Check sheet for the modelled part. Datum: model origin and axes. Units: mm. Give positions to 0.01 mm unless a question says otherwise; leave off trailing zeros. Order: outer loops, then holes, each group sorted by start corner. A loop starts at its lowest first (then second) coordinate and runs counter-clockwise, first axis right, second up. Notation, with made-up numbers: (22, 3) -> (40, 3) arc R19 ccw to (40, 37) -> close; hole circle Ø1 at (61.25, 88). An arc over 180 degrees is marked (long way). Answer in a Markdown table with one row per item. Add a question column.
(1) Cross-section at B-B (x = 4.75). Record the cut outline in (y, z), then the cut area to 3 significant figures.
(2) Thickness scan on L1, parallel to Y at x = 6, z = 3.75; L2, parallel to Z at x = -1.75, y = 1.85; L3, parallel to Z at x = -1.5, y = 2.9. Record the ranges inside material, lowest first. Write a range as [from, to].
(3) Cross-section at A-A (y = 4.15). Record the cut outline in (x, z).
(4) Go/stop test with flat-tipped pins: pin 1 (5 mm diameter, centred on x = 0, z = 4, fed in from -Y); pin 2 (1 mm diameter, centred on x = 1.5, y = 2, fed in from -Z); pin 3 (1.5 mm diameter, centred on x = 0.5, z = -4.5, fed in from -Y). Record where each tip stops, or that it passes through.
```python
from build123d import *

# Parameters (mm, degrees)
SKETCH1_R           = 4
BOSS_EXTRUDE1_DEPTH = 5.5
BOSS_EXTRUDE2_DEPTH = 2
FILLET3_R           = 3


with BuildPart() as part:
    # Sketch1 → Boss-Extrude1 (new body)
    with BuildSketch(Plane(origin=(0, 0, 0), x_dir=(1, 0, 0), z_dir=(0, 1, 0))):
        Circle(SKETCH1_R)
    extrude(amount=BOSS_EXTRUDE1_DEPTH)

    # Sketch2 → Boss-Extrude2 (add)
    with BuildSketch(Plane(origin=(0, 5.5, 0), x_dir=(1, 0, 0), z_dir=(0, 1, 0))):
        Polygon((0.772583445, -8.200189926), (7.3705827, -3.676208734), (-0.772583445, 8.200189926), (-7.3705827, 3.676208734), align=None)
    extrude(amount=-BOSS_EXTRUDE2_DEPTH)

    # Fillet3
    fillet3_edges = [part.edges().sort_by_distance(p)[0] for p in [
        (-4, 0, 0),
    ]]
    fillet(fillet3_edges, radius=FILLET3_R)


solid = part.part
```
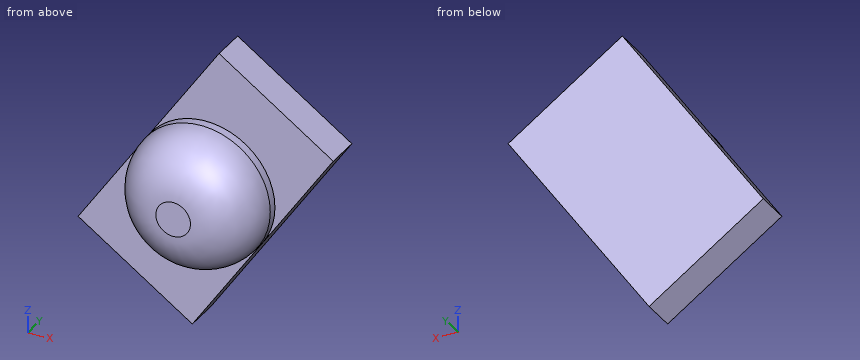
Answer below:
| question | item | result |
|---|---|---|
| 1 | outline | (3.5, -0.15) -> (5.5, -0.15) -> (5.5, 5.47) -> (3.5, 5.47) -> close |
| 1 | area | 11.2 mm² |
| 2 | L1 | y = [3.5, 5.5] |
| 2 | L2 | z = [-3.34, 3.34] |
| 2 | L3 | z = [-3.71, 3.71] |
| 3 | outline | (-7.37, -3.68) -> (-0.77, -8.2) -> (7.37, 3.68) -> (0.77, 8.2) -> close |
| 4 | pin 1 | stops at y = 0.04 |
| 4 | pin 2 | stops at z = -3.76 |
| 4 | pin 3 | stops at y = 1.87 |
